Build history of the part. All positions in model axes, mm. A direction names the side the tool comes from. Give positions to 0.01 mm unless a question says otherwise; leave off trailing zeros. Write each loop counter-clockwise with the first axis right and the second up, starting at its lowest first coordinate (ties: lowest second). Pieces come first, ordered by that corner, then holes. Notation, with made-up numbers: M 46,8 L 54,8 A11 cw 54,27 Z; hole C 18.5,-3.75 d4. An arc over 180 degrees is marked long. Return JSON: item names as keys, results as strings. Group by question number.
Q1. Band-saw the part on B-B, the plane z = 0.5. Count the separate pieces of the cut face and the enclosed holes in it, then the cut area to 3 significant figures.
Q2. Wall check: probe 1 along Y at (x, z) = (-15.25, 1); probe 2 along Y at (x, z) = (-27.5, 0.65); probe 3 along Y at (x, z) = (-14, 0.6). Give the ranges that are in metal, low to high.
Q3. Pull direction X, two halves, no side cores. Call faces 3 (the flat face through (-1, 1, 0)), 4 (the cylindrical face through (-34.06, -33.82, 0.99)), 5 (the flat face through (-13.215, -24.529, 0.986)), 6 (the cylindrical face through (-24.57, -0.35, 0.99)): +X half, -X half, draft (parallel to the pull), parting line (faces both ways), or undercut.
Q4. Tool access for faces 1 (the flat face through (12.948, 24.262, 0.986)), 2 (the cylindrical face through (-27.36, 26.51, 0.99)): list every direction of +Z, -Z, +X, -X, +Y, -Y with a clear straight run to the whole face (end or side of a thin tool).
Q5. Band-saw the part on D-D, the plane y = 3.5. Give the cut face in (x, z), then the cut area to 3 significant figures.
Q6. Band-saw the part on A-A, the plane x = -15.5. Give the cut face in (y, z), then the cut area to 3 significant figures.
Q7. Flat gauge pins, fed straight in: pin 1 Ø2.5 at (x, y) = (-28.28, -28.28) entering from -Z; pin 2 Ø1 at (y, z) = (7.5, 1.5) entering from -X. Where does each tip first touch, or does it go through?
Q8. Band-saw the part on C-C, the plane y = 21.5. Give the cut face in (x, z), then the cut area to 3 significant figures.
from build123d import *

# Parameters (mm, degrees)
SKETCH_R      = 2
SKETCH_R_2    = 1.5
EXTRUDE_DEPTH = 2


with BuildPart() as part:
    # Sketch → Extrude (new body)
    with BuildSketch(Plane.XY):
        with BuildLine():
            ThreePointArc((-22.627417, 33.941125), (-33.941125, 33.941125), (-33.941125, 22.627417))
            ThreePointArc((-33.941125, -22.627417), (-24.568542, 0), (-33.941125, 22.627417))
            ThreePointArc((-33.941125, -22.627417), (-33.941125, -33.941125), (-22.627417, -33.941125))
            Line((-22.627417, -33.941125), (-3.535534, -14.849242))
            ThreePointArc((3.535534, -14.849242), (0, -13.384776), (-3.535534, -14.849242))
            Line((3.535534, -14.849242), (22.627417, -33.941125))
            ThreePointArc((22.627417, -33.941125), (33.941125, -33.941125), (33.941125, -22.627417))
            ThreePointArc((33.941125, 22.627417), (24.568542, 0), (33.941125, -22.627417))
            ThreePointArc((33.941125, 22.627417), (33.941125, 33.941125), (22.627417, 33.941125))
            Line((3.535534, 14.849242), (22.627417, 33.941125))
            ThreePointArc((-3.535534, 14.849242), (0, 13.384776), (3.535534, 14.849242))
            Line((-22.627417, 33.941125), (-3.535534, 14.849242))
        make_face()
        with Locations((28.284271, 28.284271)):
            Circle(SKETCH_R, mode=Mode.SUBTRACT)
        with Locations((28.284271, -28.284271)):
            Circle(SKETCH_R, mode=Mode.SUBTRACT)
        with Locations((-28.284271, -28.284271)):
            Circle(SKETCH_R, mode=Mode.SUBTRACT)
        with Locations((-28.284271, 28.284271)):
            Circle(SKETCH_R, mode=Mode.SUBTRACT)
        with Locations((15.25, 15.25)):
            Circle(SKETCH_R_2, mode=Mode.SUBTRACT)
        with Locations((-15.25, 15.25)):
            Circle(SKETCH_R_2, mode=Mode.SUBTRACT)
        with Locations((-15.25, -15.25)):
            Circle(SKETCH_R_2, mode=Mode.SUBTRACT)
        with Locations((15.25, -15.25)):
            Circle(SKETCH_R_2, mode=Mode.SUBTRACT)
    extrude(amount=EXTRUDE_DEPTH)


solid = part.part
From the geometry:
{
 "1": {"separate pieces": "1", "enclosed holes": "8", "area": "3,080 mm^2"},
 "2": {"probe 1": "y = -26.56 to -16.75, -13.75 to 13.75, 16.75 to 26.56", "probe 2": "y = -36.25 to -30.12, -26.44 to -13.38, 13.38 to 26.44, 30.12 to 36.25", "probe 3": "y = -25.31 to -16.08, -14.42 to 14.42, 16.08 to 25.31"},
 "3": {"face 3": "draft", "face 4": "undercut", "face 5": "undercut", "face 6": "-X half"},
 "4": {"face 1": "+Z, -Z, +Y", "face 2": "+Z, -Z"},
 "5": {"outline": "M -24.76,0 L 24.76,0 L 24.76,2 L -24.76,2 Z", "area": "99.0 mm^2"},
 "6": {"outline": "M -26.81,0 L -16.73,0 L -16.73,2 L -26.81,2 Z; M -13.77,0 L 13.77,0 L 13.77,2 L -13.77,2 Z; M 16.73,0 L 26.81,0 L 26.81,2 L 16.73,2 Z", "area": "95.4 mm^2"},
 "7": {"pin 1": "passes through", "pin 2": "stops at x = -25.58"},
 "8": {"outline": "M -32.87,0 L -10.19,0 L -10.19,2 L -32.87,2 Z; M 10.19,0 L 32.87,0 L 32.87,2 L 10.19,2 Z", "area": "90.7 mm^2"}
}
